from build123d import *

# Parameters (mm, degrees)
F0_W     = 4
F0_H     = 4
F0_H_2   = 6
F1_DEPTH = 90
F2_W     = 80
F2_H     = 6.35
F3_DEPTH = 25
F4_R     = 3.17499


# Not quite as in the source:
# - a fillet or chamfer is up to 0.001 mm smaller than in the source, because OpenCascade refuses the exact size


with BuildPart() as f1:
    # F0 (on Front) → F1 (new body)
    with BuildSketch(Plane.XZ):
        with Locations((-13, 27)):
            Rectangle(F0_W, F0_H)
        with Locations((-13, 22)):
            Rectangle(F0_W, F0_H_2)
        Polygon((-11, 19), (-15, 19), (-15, 0), (-2, 0), (-2, -43.675), (-20, -43.675), (-20, -47.675), (0, -47.675), (0, 0), (0, 4), (-11, 4), align=None)
    extrude(amount=F1_DEPTH)

    # F2 (on face) → F3 (cut)
    with BuildSketch(Plane(origin=(-15, 0, 0), x_dir=(0, -1, 0), z_dir=(-1, 0, 0))):
        with Locations((45, 19)):
            Rectangle(F2_W, F2_H)
    extrude(amount=-F3_DEPTH, mode=Mode.SUBTRACT)

    # F4 (radius 3.175 in the source; OpenCascade refuses exactly that, so slightly less here)
    f4_edges = [f1.edges().sort_by_distance(p)[0] for p in [
        (-13, 0, 29),
        (-13, -90, 29),
        (-11, -45, 4),
        (-15, -45, 0),
        (-20, 0, -45.675),
        (-20, -90, -45.675),
        (-13, -85, 22.175),
        (-13, -85, 15.825),
        (-13, -5, 15.825),
        (-13, -5, 22.175),
        (-2, -45, -43.675),
        (-2, -45, 0),
    ]]
    fillet(f4_edges, radius=F4_R)

    # F5: F1 across plane


with BuildPart() as f1_1:
    add(f1.part)
    add(f1.part.mirror(Plane.YZ))


solid = f1_1.part
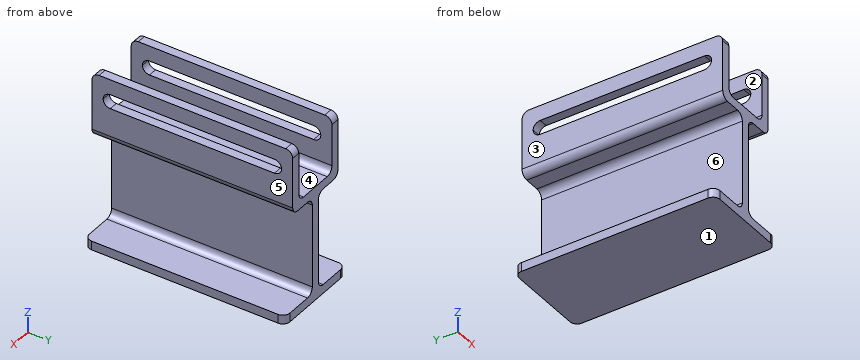
Could you check a few things on this model? Use its own coordinates, in mm. Face numbers are marked on the shaded views. A direction names the side the tool comes from. Coordinates: 2 decimals unless noted, no trailing zeros. Order: outer loops, then holes, each group sorted by start corner. A loop starts at its lowest first (then second) coordinate and runs counter-clockwise, first axis right, second up. Notation, with made-up numbers: (19, -31.75) -> (39, -31.75) arc R28 cw to (39, -12.75) -> close; hole circle Ø10 at (76, -9.5). An arc over 180 degrees is marked (long way). One line per item, written item: value. Start each with the question number.
1) Imagine slicing it at C-C on z = 17. List the corners of the cut face in (x, y) for me.
2) We'd pull the mould along X, two halves only. Please class the marked faces 1, 2 and 3: +X half, -X half, draft (parallel to the pull), parting line (faces both ways), or undercut.
3) Imagine slicing it at A-A on y = -35.5. Count the separate pieces of the cut face and the enclosed holes in it, plus the area to 3 significant figures.
4) I'm going to push flat-ended pins straight in: pin 1 (13 mm diameter, centred on y = -67, z = 16, fed in from -X); pin 2 (18.5 mm diameter, centred on y = -38.5, z = -15, fed in from +X); pin 3 (12 mm diameter, centred on y = -50.5, z = -8, fed in from +X). Where does each tip first touch, or does it pass through?
5) If I drill on L1, parallel to Z at x = 8, y = -77.5 (3 decimals); L2, parallel to X at y = -28, z = -35; L3, parallel to Z at x = -2.5, y = -53 (3 decimals), over which ranges is the centre line in solid material (lowest first)? Write a range as [from, to].
6) Which directions (+Z, -Z, +X, -X, +Y, -Y) give clear straight access to the entire face, cutting with the end or side of a thin tool? Please do the marked faces 4, 5 and 6.
7) Imagine slicing it at D-D on x = 9. List the corners of the cut face in (y, z) for me (3 decimals), plus the area to 3 significant figures.
Answer list:
1. outline: (-15, -90) -> (-11, -90) -> (-11, -84.29) -> (-15, -84.29) -> close; (-15, -5.71) -> (-11, -5.71) -> (-11, 0) -> (-15, 0) -> close; (11, -90) -> (15, -90) -> (15, -84.29) -> (11, -84.29) -> close; (11, -5.71) -> (15, -5.71) -> (15, 0) -> (11, 0) -> close
2. face 1: draft
2. face 2: undercut
2. face 3: -X half
3. separate pieces: 3
3. enclosed holes: 0
3. area: 613 mm2
4. pin 1: stops at x = -15
4. pin 2: stops at x = 2
4. pin 3: stops at x = 2.23
5. L1: z = [-47.675, -43.675], [0, 4.005]
5. L2: x = [-2, 2]
5. L3: z = [-47.675, -42.21], [-1.465, 4]
6. face 4: +Z, +Y, -Y
6. face 5: +Z, +X, +Y, -Y
6. face 6: -X, +Y, -Y
7. outline: (-90, -47.675) -> (0, -47.675) -> (0, -43.675) -> (-90, -43.675) -> close; (-90, 0) -> (0, 0) -> (0, 4.225) -> (-90, 4.225) -> close
7. area: 740 mm2
